from build123d import *

# Parameters (mm, degrees)
F1_DEPTH      = 10
F2_R          = 105
F3_DEPTH      = 4
F3_DEPTH_BACK = 4
F4_R          = 2.5
F6_DEPTH      = 4
F8_START      = -2
F8_DEPTH      = 16
F9_W          = 140
F9_H          = 40
F10_DEPTH     = 0.5
F11_R         = 5


with BuildPart() as f1:
    # F0 (on Front) → F1 (new body, symmetric)
    with BuildSketch(Plane.XZ):
        with BuildLine():
            Line((-70, 50.7738371067), (-70, 0))
            Line((-70, 0), (70, 0))
            Line((70, 0), (70, 50.7738371067))
            ThreePointArc((70, 50.7738371067), (0, 20), (-70, 50.7738371067))
        make_face()
    extrude(amount=F1_DEPTH, both=True)

    # F2 (on Front) → F3 (cut, two sides)
    with BuildSketch(Plane.XZ) as f3_sk:
        with Locations((0, 115)):
            Circle(F2_R)
    extrude(amount=-F3_DEPTH, mode=Mode.SUBTRACT)
    extrude(f3_sk.sketch, amount=F3_DEPTH_BACK, mode=Mode.SUBTRACT)

    # F4
    f4_edges = [f1.edges().sort_by_distance(p)[0] for p in [
        (-70, 7, 50.773837),
        (-70, -7, 50.773837),
        (70, 7, 50.773837),
        (70, -7, 50.773837),
    ]]
    fillet(f4_edges, radius=F4_R)

    # F5 (on Front) → F6 (cut, symmetric)
    with BuildSketch(Plane.XZ):
        with BuildLine():
            Line((-62, 43.0208363483), (-62, 15.899041377))
            ThreePointArc((-62, 15.899041377), (-50, 3.899041377), (-38, 15.899041377))
            Line((-38, 15.899041377), (-38, 43.0208363483))
            Line((-38, 43.0208363483), (-62, 43.0208363483))
        make_face()
        with BuildLine():
            ThreePointArc((38, 15.899041377), (50, 3.899041377), (62, 15.899041377))
            Line((62, 15.899041377), (62, 43.0208363483))
            Line((62, 43.0208363483), (38, 43.0208363483))
            Line((38, 43.0208363483), (38, 15.899041377))
        make_face()
    extrude(amount=F6_DEPTH, both=True, mode=Mode.SUBTRACT)

    # F7 (on face) → F8 (cut)
    with BuildSketch(Plane.XZ.offset(10).offset(F8_START)):
        with BuildLine():
            Line((-54, 36.8399078813), (-54, 15.899041377))
            ThreePointArc((-54, 15.899041377), (-50, 11.899041377), (-46, 15.899041377))
            Line((-46, 15.899041377), (-46, 36.8399078813))
            Line((-46, 36.8399078813), (-54, 36.8399078813))
        make_face()
        with BuildLine():
            ThreePointArc((46, 15.899041377), (50, 11.899041377), (54, 15.899041377))
            Line((54, 15.899041377), (54, 36.8399078813))
            Line((54, 36.8399078813), (46, 36.8399078813))
            Line((46, 36.8399078813), (46, 15.899041377))
        make_face()
    extrude(amount=-F8_DEPTH, mode=Mode.SUBTRACT)

    # F9 (on Top) → F10 (join, symmetric)
    with BuildSketch(Plane.XY):
        Rectangle(F9_W, F9_H)
    extrude(amount=F10_DEPTH, both=True)

    # F11
    f11_edges = [f1.edges().sort_by_distance(p)[0] for p in [
        (-70, -20, 0),
        (70, -20, 0),
        (70, 20, 0),
        (-70, 20, 0),
    ]]
    fillet(f11_edges, radius=F11_R)


solid = f1.part
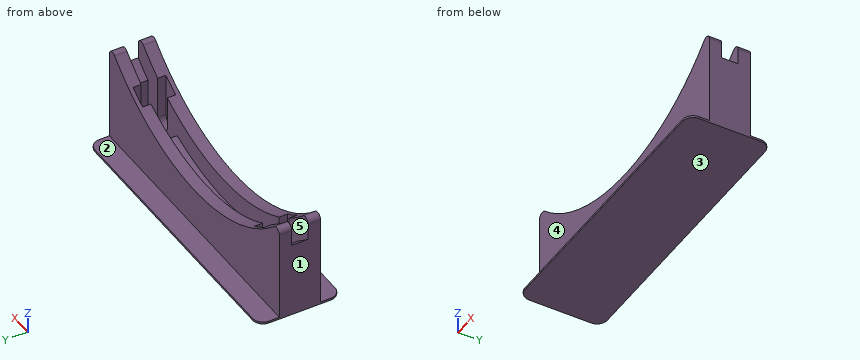
Geometry check sheet. Reference: the model listing, model coordinates, mm. Face numbers are marked on the shaded views. A direction names the side the tool comes from. Give positions to 0.01 mm unless a question says otherwise; leave off trailing zeros. Write each loop counter-clockwise with the first axis right and the second up, starting at its lowest first coordinate (ties: lowest second). Pieces come first, ordered by that corner, then holes. Notation, with made-up numbers: M 6.5,74.5 L 27.5,74.5 A37 ccw 27.5,112.5 Z; hole C 65,68 d1. An arc over 180 degrees is marked long. Answer as CSV lines item,"result". Start each with the question number.
Q1. Go/stop test with flat-tipped pins: pin 1 (12 mm diameter, centred on x = 38.5, y = -13.5, fed in from +Z); pin 2 (23.5 mm diameter, centred on x = -22, z = 25, fed in from -Y); pin 3 (5 mm diameter, centred on x = 22.5, y = -5, fed in from +Z); pin 4 (5 mm diameter, centred on y = -12, z = 29, fed in from +X). Record where each tip stops, or that it passes through.
Q2. Section check B-B, the plane y = 6. Record the cut outline in (x, z), then the cut area to 3 significant figures.
Q3. Release check for a two-part mould opening along Y. For the marked faces 3, 4 and 5 record: pulls with the +Y half, pulls with the -Y half, needs draft (parallel to the pull), parting line crosses it, or undercut.
Q4. Section check A-A, the plane x = -50. Record the cut outline in (y, z).
Q5. Section check C-C, the plane x = 22. Record the cut outline in (y, z).
Q6. Tool access check on the marked faces 1 and 2. Record the directions out of +Z, -Z, +X, -X, +Y, -Y that give a thin tool (end or side, any length) a straight path to the whole face; none if there is none.
Q7. Material ranges on L1, parallel to X at y = 6, z = 43; L2, parallel to X at y = 7, z = 15.5; L3, parallel to X at y = 5.5, z = 27, recorded low to high.
Geometry says:
1,pin 1,"z = 30.48"
1,pin 2,"y = -10"
1,pin 3,"z = 23.35"
1,pin 4,"x = 70"
2,outline,"M -70,-0.5 L 70,-0.5 L 70,44.64 A2.5 ccw 65.77,46.45 A95 cw 54,36.84 L 54,15.9 A4 cw 46,15.9 L 46,31.88 A95 cw -46,31.88 L -46,15.9 A4 cw -54,15.9 L -54,36.84 A95 cw -65.77,46.45 A2.5 ccw -70,44.64 Z"
2,area,"3,840 mm^2"
3,face 3,"needs draft"
3,face 4,"pulls with the -Y half"
3,face 5,"undercut"
4,outline,"M -20,-0.5 L 20,-0.5 L 20,0.5 L 10,0.5 L 10,34.22 L 8,34.22 L 8,11.9 L 4,11.9 L 4,3.9 L -4,3.9 L -4,11.9 L -8,11.9 L -8,34.22 L -10,34.22 L -10,0.5 L -20,0.5 Z"
5,outline,"M -20,-0.5 L 20,-0.5 L 20,0.5 L 10,0.5 L 10,22.58 L 4,22.58 L 4,12.33 L -4,12.33 L -4,22.58 L -10,22.58 L -10,0.5 L -20,0.5 Z"
6,face 1,"+Z, -Z, -X, +Y, -Y"
6,face 2,"+Z, +X, -X, +Y"
7,L1,"-70 to -61.98, 61.98 to 70"
7,L2,"-70 to -53.98, -46.02 to 46.02, 53.98 to 70"
7,L3,"-70 to -54, -46 to -35.79, 35.79 to 46, 54 to 70"
